Verification items for the finished model (mm, model axes). Coordinates: 2 decimals unless noted, no trailing zeros. Write each loop counter-clockwise with the first axis right and the second up, starting at its lowest first coordinate (ties: lowest second). Pieces come first, ordered by that corner, then holes. Notation, with made-up numbers: M -4,68 L 2,68 A37 cw 2,104 Z; hole C 89,76 d4. An arc over 180 degrees is marked long. Answer in a Markdown table with one row per item.
from build123d import *

# Parameters (mm, degrees)
F0_W        = 38.1
F0_H        = 3.0988
F1_DEPTH    = 11.43
F3_T1_DEPTH = 61.4886973558
F4_DEPTH    = 25.4


# Not quite as in the source:
# - a fillet or chamfer that OpenCascade refuses, or shapes differently, is made with other operations: its cross-section is extruded or revolved along the edge and cut away or added


with BuildPart() as f1:
    # F0 (on Top) → F1 (new body)
    with BuildSketch(Plane.XY):
        with Locations((0, 1.5494)):
            Rectangle(F0_W, F0_H)
    extrude(amount=F1_DEPTH)

    # F3: fillet of radius 5.08 on 1 edges, made by hand

    # F3_s2 → F3_t1 (cut)
    with BuildSketch(Plane.YZ.offset(-30.7443486779)):
        with BuildLine():
            ThreePointArc((3.0988, 6.7522605288), (2.2538263281, 9.5577822272), (0, 11.43))
            Line((0, 11.43), (3.0988, 11.43))
            Line((3.0988, 11.43), (3.0988, 6.7522605288))
        make_face()
    extrude(amount=F3_T1_DEPTH, mode=Mode.SUBTRACT)

    # F2 (on face) → F4 (cut)
    with BuildSketch(Plane.XZ):
        Polygon((-15.875, 10.2462954744), (-15.1915878735, 11.43), (-16.5584121265, 11.43), align=None)
        Polygon((-4.9582643893, 11.43), (-6.4717356107, 11.43), (-5.715, 10.1192954744), align=None)
        Polygon((5.1284121265, 11.43), (3.7615878735, 11.43), (4.445, 10.2462954744), align=None)
        Polygon((16.4850886423, 11.43), (15.2649113577, 11.43), (15.875, 10.3732954744), align=None)
    extrude(amount=-F4_DEPTH, mode=Mode.SUBTRACT)


solid = f1.part
1) Sectioned sample at A-A (z = 10.75). Record the cut outline in (x, y).
Response values:
| item | result |
|---|---|
| outline | M -19.05,0 L -16.17,0 L -16.17,1.15 L -19.05,1.15 Z; M -15.58,0 L -6.08,0 L -6.08,1.15 L -15.58,1.15 Z; M -5.35,0 L 4.15,0 L 4.15,1.15 L -5.35,1.15 Z; M 4.74,0 L 15.66,0 L 15.66,1.15 L 4.74,1.15 Z; M 16.09,0 L 19.05,0 L 19.05,1.15 L 16.09,1.15 Z |
2) Sectioned sample at B-B (y = 1.25). Record the cut outline in (x, z) (3 decimals), then the cut area to 3 significant figures.
Response values:
| item | result |
|---|---|
| outline | M -19.05,0 L 19.05,0 L 19.05,10.672 L 16.048,10.672 L 15.875,10.373 L 15.702,10.672 L 4.691,10.672 L 4.445,10.246 L 4.199,10.672 L -5.396,10.672 L -5.715,10.119 L -6.034,10.672 L -15.629,10.672 L -15.875,10.246 L -16.121,10.672 L -19.05,10.672 Z |
| area | 406 mm² |
3) Sectioned sample at C-C (x = 0). Record the cut outline in (y, z), then the cut area to 3 significant figures.
Response values:
| item | result |
|---|---|
| outline | M 0,0 L 3.1,0 L 3.1,6.75 A5.08 ccw 0,11.43 Z |
| area | 31.4 mm² |
4) Sectioned sample at D-D (z = 7.5). Record the cut outline in (x, y), then the cut area to 3 significant figures.
Response values:
| item | result |
|---|---|
| outline | M -19.05,0 L 19.05,0 L 19.05,3.04 L -19.05,3.04 Z |
| area | 116 mm² |
5) Thickness scan on L1, parallel to Y at x = -15, z = 10.5; L2, parallel to Y at x = 2.5, z = 10.75; L3, parallel to Z at x = 2, y = 1.85. Record the ranges inside material, lowest first. Write a range as [from, to].
Response values:
| item | result |
|---|---|
| L1 | y = [0, 1.45] |
| L2 | y = [0, 1.15] |
| L3 | z = [0, 10.09] |
6) Depth check by flat-ended pin: pin 1 (1.5 mm diameter, centred on x = 12.5, y = 2.5, fed in from +Z). Enter the tip coordinate at first touch or a pass-through.
Response values:
| item | result |
|---|---|
| pin 1 | stops at z = 10.2 |
7) Release check for a two-part mould opening along X. For faces 1 (the face through (19.05, 2, 6)), 2 (the face through (0, 2, 0)), 3 (the face through (-19.05, 2, 6)), 4 (the face through (4.706, 0.652, 10.698)) record: +X half, -X half, draft (parallel to the pull), parting line (faces both ways), or undercut.
Response values:
| item | result |
|---|---|
| face 1 | +X half |
| face 2 | draft |
| face 3 | -X half |
| face 4 | undercut |
